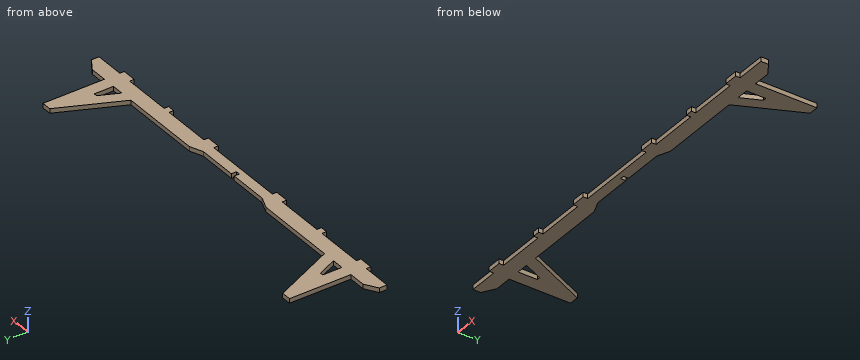
from build123d import *

# Parameters (mm, degrees)
BOSS_EXTRUDE1_DEPTH = 3.5


with BuildPart() as part:
    # Sketch1 → Boss-Extrude1 (new body)
    with BuildSketch(Plane.XY):
        Polygon((75, 12), (96.871, 60), (104.371, 60), (104.371, 12), (108.371, 12), (117.871, 12), (127.371, 6), (127.371, 0), (112.371, 0), (104.371, 0), (104.371, -3.5), (93.371, -3.5), (93.371, 0), (55.135445, 0), (55.135445, -3.5), (49.535445, -3.5), (49.535445, 0), (11, 0), (11, -3.5), (0, -3.5), (0, 0), (-65, 0), (-65, -3.5), (-76, -3.5), (-76, 0), (-114.535445, 0), (-114.535445, -3.5), (-120.135445, -3.5), (-120.135445, 0), (-158.371, 0), (-158.371, -3.5), (-169.371, -3.5), (-169.371, 0), (-177.371, 0), (-192.371, 0), (-192.371, 6), (-182.871, 12), (-173.371, 12), (-169.371, 12), (-169.371, 60), (-161.871, 60), (-140, 12), (-75, 12), (-65, 8), (-34.1, 8), (-34.1, 4), (-30.9, 4), (-30.9, 8), (0, 8), (10, 12), align=None)
        Polygon((85, 12), (91.8346875, 27), (94.371, 27), (94.371, 12), align=None, mode=Mode.SUBTRACT)
        Polygon((-150, 12), (-159.371, 12), (-159.371, 27), (-156.8346875, 27), align=None, mode=Mode.SUBTRACT)
    extrude(amount=BOSS_EXTRUDE1_DEPTH)


solid = part.part
The listing builds one solid part. Answer for the finished solid, in the listing's coordinates (mm). Give positions to 0.01 mm unless a question says otherwise; leave off trailing zeros. Loops run counter-clockwise (first coordinate to the right, second up) from the corner with the lowest first, then second, coordinate; pieces in that order, holes last. Notation, with made-up numbers: (-31.75, -29.75) - (-15.75, -29.75) arc R33 cw to (-15.75, 4.25) - close; hole circle Ø9 at (-24, 81.25). An arc over 180 degrees is marked (long way). Answer as a JSON object with one key per item and string values.
1. Flat-ended cylindrical pins translate along their axes: pin 1 Ø1 at (x, z) = (69, 2) entering from -Y; pin 2 Ø1.6 at (x, z) = (-33, 1.5) entering from +Y; pin 3 Ø1 at (y, z) = (-2.5, 1.5) entering from -X. Find the tip coordinate at first contact, or state that the pin passes through.
Determined:
{"pin 1": "y = 0", "pin 2": "y = 4", "pin 3": "x = -169.37"}
2. A cutting plane is placed at A-A (y = 34). Write down the section's boundary in (x, z), then the cut area to 3 significant figures.
Determined:
{"outline": "(-169.37, 0) - (-150.02, 0) - (-150.02, 3.5) - (-169.37, 3.5) - close; (85.02, 0) - (104.37, 0) - (104.37, 3.5) - (85.02, 3.5) - close", "area": "135 mm²"}
3. A cutting plane is placed at D-D (z = 2.65). Give the number of separate pieces and of enclosed holes in the cut face, then the cut area to 3 significant figures.
Determined:
{"separate pieces": "1", "enclosed holes": "2", "area": "5,250 mm²"}
4. Find the intervals of material crossed by L1, parallel to Y at x = 39, z = 2.15; L2, parallel to X at y = 4.5, z = 0.2; L3, parallel to Y at x = -46.5, z = 0.95, in increasing order. Write a range as [from, to].
Determined:
{"L1": "[0, 12]", "L2": "[-192.37, -34.1], [-30.9, 127.37]", "L3": "[0, 8]"}
5. A cutting plane is placed at B-B (y = 22). Write down the section's boundary in (x, z).
Determined:
{"outline": "(-169.37, 0) - (-159.37, 0) - (-159.37, 3.5) - (-169.37, 3.5) - close; (-154.56, 0) - (-144.56, 0) - (-144.56, 3.5) - (-154.56, 3.5) - close; (79.56, 0) - (89.56, 0) - (89.56, 3.5) - (79.56, 3.5) - close; (94.37, 0) - (104.37, 0) - (104.37, 3.5) - (94.37, 3.5) - close"}
6. A cutting plane is placed at C-C (x = 7). Write down the section's boundary in (y, z).
Determined:
{"outline": "(-3.5, 0) - (10.8, 0) - (10.8, 3.5) - (-3.5, 3.5) - close"}
